Geometry: final body of the model. Coordinates: model frame, mm. A direction names the side the tool comes from. Give positions to 0.01 mm unless a question says otherwise; leave off trailing zeros. Loops run counter-clockwise (first coordinate to the right, second up) from the corner with the lowest first, then second, coordinate; pieces in that order, holes last. Notation, with made-up numbers: (61, -34) -> (77, -34) arc R7 ccw to (77, -23) -> close; hole circle Ø1 at (89, 57). An arc over 180 degrees is marked (long way). One line per item, written item: value. Start each with the question number.
from build123d import *

# Parameters (mm, degrees)
SKETCH2_W           = 75
SKETCH2_H           = 25
BOSS_EXTRUDE1_DEPTH = 3
BOSS_EXTRUDE2_DEPTH = 30
SKETCH5_W           = 6
SKETCH5_H           = 30
BOSS_EXTRUDE3_DEPTH = 8
SKETCH6_W           = 6
SKETCH6_H           = 30
BOSS_EXTRUDE4_DEPTH = 8
SKETCH8_R           = 1.75
CUT_EXTRUDE1_DEPTH  = 8
CUT_EXTRUDE2_DEPTH  = 6
FILLET1_R           = 5
FILLET2_R           = 5
SKETCH13_W          = 6
SKETCH13_H          = 2
CUT_EXTRUDE3_DEPTH  = 36
FILLET3_R           = 0.5


with BuildPart() as part:
    # Sketch2 → Boss-Extrude1 (new body)
    with BuildSketch(Plane(origin=(0, 0, 0), x_dir=(1, 0, 0), z_dir=(0, 1, 0))):
        with Locations((0, 12.5)):
            Rectangle(SKETCH2_W, SKETCH2_H)
    extrude(amount=BOSS_EXTRUDE1_DEPTH)

    # Sketch3 → Boss-Extrude2 (add)
    with BuildSketch(Plane(origin=(0, 3, 0), x_dir=(1, 0, 0), z_dir=(0, 1, 0))):
        Polygon((-35.5, 0), (-35.5, 23), (35.5, 23), (35.5, 0), (37.5, 0), (37.5, 25), (-37.5, 25), (-37.5, 0), align=None)
    extrude(amount=BOSS_EXTRUDE2_DEPTH)

    # Sketch5 → Boss-Extrude3 (add)
    with BuildSketch(Plane.ZY.offset(37.5)):
        with Locations((-3, 18)):
            Rectangle(SKETCH5_W, SKETCH5_H)
    extrude(amount=BOSS_EXTRUDE3_DEPTH)

    # Sketch6 → Boss-Extrude4 (add)
    with BuildSketch(Plane(origin=(37.5, 0, 0), x_dir=(0, 0, -1), z_dir=(1, 0, 0))):
        with Locations((3, 18)):
            Rectangle(SKETCH6_W, SKETCH6_H)
    extrude(amount=BOSS_EXTRUDE4_DEPTH)

    # Sketch8 → Cut-Extrude1 (cut)
    with BuildSketch(Plane.XY):
        with Locations((-42.5, 29)):
            Circle(SKETCH8_R)
        with Locations((42.5, 29)):
            Circle(SKETCH8_R)
        with Locations((-42.5, 19)):
            Circle(SKETCH8_R)
        with Locations((-42.5, 9)):
            Circle(SKETCH8_R)
        with Locations((42.5, 19)):
            Circle(SKETCH8_R)
        with Locations((42.5, 9)):
            Circle(SKETCH8_R)
    extrude(amount=-CUT_EXTRUDE1_DEPTH, mode=Mode.SUBTRACT)

    # Sketch12 → Cut-Extrude2 (cut)
    with BuildSketch(Plane.XY):
        Polygon((-35.5, 33), (-37, 33), (-37, 1.5), (37, 1.5), (37, 33), (35.5, 33), (35.5, 3), (-35.5, 3), align=None)
    extrude(amount=-CUT_EXTRUDE2_DEPTH, mode=Mode.SUBTRACT)

    # Fillet1
    # the kernel refuses this fillet: 5 mm, written as the material it adds along each edge
    with BuildSketch(Plane(origin=(-37.5, 33, -6), x_dir=(0, 0, -1), z_dir=(0, -1, 0))) as fillet1_piece_1_section:
        with BuildLine():
            CenterArc((FILLET1_R, -FILLET1_R), FILLET1_R, 90, 90)
            Line((0, -FILLET1_R), (0, 0))
            Line((0, 0), (FILLET1_R, 0))
        make_face()
    fillet1_piece_1 = extrude(amount=30, mode=Mode.PRIVATE)
    fillet1_piece_1 = fillet1_piece_1 - Plane(origin=(-42.5, 29, -7.147283254), x_dir=(1, 0, 0), z_dir=(0, 0, 1)) * Cylinder(1.75, 80, mode=Mode.PRIVATE)
    fillet1_piece_1 = fillet1_piece_1 - Plane(origin=(-42.5, 19, -7.147283254), x_dir=(1, 0, 0), z_dir=(0, 0, 1)) * Cylinder(1.75, 80, mode=Mode.PRIVATE)
    fillet1_piece_1 = fillet1_piece_1 - Plane(origin=(-42.5, 9, -7.147283254), x_dir=(1, 0, 0), z_dir=(0, 0, 1)) * Cylinder(1.75, 80, mode=Mode.PRIVATE)
    add(fillet1_piece_1)

    # Fillet2
    # the kernel refuses this fillet: 5 mm, written as the material it adds along each edge
    with BuildSketch(Plane(origin=(37.5, 33, -6), x_dir=(1, 0, 0), z_dir=(0, -1, 0))) as fillet2_piece_1_section:
        with BuildLine():
            CenterArc((FILLET2_R, -FILLET2_R), FILLET2_R, 90, 90)
            Line((0, -FILLET2_R), (0, 0))
            Line((0, 0), (FILLET2_R, 0))
        make_face()
    fillet2_piece_1 = extrude(amount=30, mode=Mode.PRIVATE)
    fillet2_piece_1 = fillet2_piece_1 - Plane(origin=(42.5, 9, -7.147283906), x_dir=(1, 0, 0), z_dir=(0, 0, 1)) * Cylinder(1.75, 80, mode=Mode.PRIVATE)
    fillet2_piece_1 = fillet2_piece_1 - Plane(origin=(42.5, 29, -7.147283906), x_dir=(1, 0, 0), z_dir=(0, 0, 1)) * Cylinder(1.75, 80, mode=Mode.PRIVATE)
    fillet2_piece_1 = fillet2_piece_1 - Plane(origin=(42.5, 19, -7.147283906), x_dir=(1, 0, 0), z_dir=(0, 0, 1)) * Cylinder(1.75, 80, mode=Mode.PRIVATE)
    add(fillet2_piece_1)

    # Sketch13 → Cut-Extrude3 (cut)
    with BuildSketch(Plane(origin=(0, 33, 0), x_dir=(1, 0, 0), z_dir=(0, 1, 0))):
        with Locations((-42.5, 7)):
            Rectangle(SKETCH13_W, SKETCH13_H)
        with Locations((42.5, 7)):
            Rectangle(SKETCH13_W, SKETCH13_H)
    extrude(amount=-CUT_EXTRUDE3_DEPTH, mode=Mode.SUBTRACT)

    # Fillet3
    fillet3_edges = [part.edges().sort_by_distance(p)[0] for p in [
        (-35.5, 18, -23),
        (35.5, 18, -23),
    ]]
    fillet(fillet3_edges, radius=FILLET3_R)


solid = part.part
Item 1: Section C-C, the plane z = -1.5. Output: boundary loops of the cut face in (x, y), then the cut area to 3 significant figures.
Item 2: Section A-A, the plane x = -42.5. Output: boundary loops of the cut face in (y, z).
Item 3: Access query for faces 5 (the face through (-40, 18, -6)), 6 (the face through (-41, 3, -3)), 7 (the face through (40, 18, -6)), 8 (the face through (-17, 2, -6)). Directions: +Z, -Z, +X, -X, +Y, -Y. A direction counts if a zero-diameter tool reaches every point of the face in a straight line with its end or side. Return the directions, or none.
Item 4: Section D-D, the plane z = -12.75. Output: boundary loops of the cut face in (x, y).
Item 5: Ray query, line 1 along Y through (x, z) = (-42.5, -2.95); line 2 along X through (y, z) = (4, -18.25); line 3 along X through (y, z) = (12.5, -3). Return the intervals inside material, ascending. Write a range as [from, to].
Item 6: Section B-B, the plane y = 29. State how many separate pieces and enclosed holes the cut face has, then the cut area to 3 significant figures.
Item 7: Pin query (flat end, axial travel): pin 1 (16 mm diameter, centred on x = -9, y = 16.5, fed in from +Z); pin 2 (10 mm diameter, centred on x = -31, y = 21, fed in from +Z); pin 3 (5 mm diameter, centred on x = 5, z = -17, fed in from +Y); pin 4 (2 mm diameter, centred on x = -42.5, y = 29, fed in from +Z). Return the tip coordinate at first contact, or that it passes through.
Item 8: Mould query, pull axis Y, two halves, no side actions, for faces 1 (the face through (42, 3, -3)), 2 (the face through (0, 33, -24)), 3 (the face through (1, 16, -25)), 4 (the face through (-40.831, 9.526, -2.958)). Classes: pulls with the +Y half, pulls with the -Y half, needs draft (parallel to the pull), parting line crosses it, or undercut.
Geometry check:
1. outline: (-45.5, 3) -> (-37.5, 3) -> (-37.5, 0) -> (37.5, 0) -> (37.5, 3) -> (45.5, 3) -> (45.5, 33) -> (37, 33) -> (37, 1.5) -> (-37, 1.5) -> (-37, 33) -> (-45.5, 33) -> close; hole circle Ø3.5 at (-42.5, 9); hole circle Ø3.5 at (-42.5, 19); hole circle Ø3.5 at (-42.5, 29); hole circle Ø3.5 at (42.5, 9); hole circle Ø3.5 at (42.5, 19); hole circle Ø3.5 at (42.5, 29)
1. area: 566 mm2
2. outline: (3, -6) -> (7.25, -6) -> (7.25, 0) -> (3, 0) -> close; (10.75, -6) -> (17.25, -6) -> (17.25, 0) -> (10.75, 0) -> close; (20.75, -6) -> (27.25, -6) -> (27.25, 0) -> (20.75, 0) -> close; (30.75, -6) -> (33, -6) -> (33, 0) -> (30.75, 0) -> close
3. face 5: -Z, -X, +Y, -Y
3. face 6: +Z, -Z, -X, -Y
3. face 7: -Z, +X, +Y, -Y
3. face 8: +Z, +Y
4. outline: (-37.5, 0) -> (37.5, 0) -> (37.5, 33) -> (35.5, 33) -> (35.5, 3) -> (-35.5, 3) -> (-35.5, 33) -> (-37.5, 33) -> close
5. line 1: y = [3, 7.25], [10.75, 17.25], [20.75, 27.25], [30.75, 33]
5. line 2: x = [-37.5, -35.5], [35.5, 37.5]
5. line 3: x = [-45.5, -37], [37, 45.5]
6. separate pieces: 3
6. enclosed holes: 0
6. area: 287 mm2
7. pin 1: stops at z = -23
7. pin 2: stops at z = -6
7. pin 3: stops at y = 3
7. pin 4: passes through
8. face 1: pulls with the -Y half
8. face 2: pulls with the +Y half
8. face 3: needs draft
8. face 4: undercut
